Model file for the job. Use its own axes, mm. A direction names the side the tool comes from. Round coordinates to 2 decimals unless told otherwise and drop trailing zeros. Loops run counter-clockwise (first coordinate to the right, second up) from the corner with the lowest first, then second, coordinate; pieces in that order, holes last. Notation, with made-up numbers: M -29,-34.75 L -18,-34.75 A13 ccw -18,-22.75 Z; hole C 72.25,34 d5. An arc over 180 degrees is marked long. Answer in a Markdown table with one row per item.
from build123d import *

# Parameters (mm, degrees)
F0_R      = 30
F1_DEPTH  = 20
F2_R      = 4
F3_DEPTH  = 30
F4_R      = 21.9
F5_DEPTH  = 5
F6_SIZE   = 2
F7_R      = 20
F7_R_2    = 19.9
F8_DEPTH  = 42
F9_R      = 21.9
F9_R_2    = 20
F10_DEPTH = 3
F12_DEPTH = 70
F13_R     = 4
F14_DEPTH = 30.0010001


with BuildPart() as f1:
    # F0 (on Top) → F1 (new body)
    with BuildSketch(Plane.XY):
        Circle(F0_R)
    extrude(amount=F1_DEPTH)

    # F2 (on Front) → F3 (cut)
    with BuildSketch(Plane.XZ):
        with Locations((0, 10.1209855556)):
            Circle(F2_R)
    extrude(amount=F3_DEPTH, mode=Mode.SUBTRACT)

    # F4 (on face) → F5 (join)
    with BuildSketch(Plane.XY.offset(20)):
        Circle(F4_R)
    extrude(amount=F5_DEPTH)

    # F6
    f6_edges = [f1.edges().sort_by_distance(p)[0] for p in [
        (-21.9, 0, 25),
    ]]
    chamfer(f6_edges, length=F6_SIZE)

    # F7 (on face) → F8 (join)
    with BuildSketch(Plane.XY.offset(25)):
        Circle(F7_R)
        Circle(F7_R_2, mode=Mode.SUBTRACT)
        Circle(F7_R_2)
    extrude(amount=F8_DEPTH)

    # F9 (on face) → F10 (join)
    with BuildSketch(Plane.XY.offset(67)):
        Circle(F9_R)
        Circle(F9_R_2, mode=Mode.SUBTRACT)
        Circle(F9_R_2)
    extrude(amount=F10_DEPTH)

    # F11 (on face) → F12 (cut)
    with BuildSketch(Plane.XY.offset(70)):
        with BuildLine():
            Line((18.9816207227, 3.9478135966), (16.0207605252, 3.9478135966))
            ThreePointArc((16.0207605252, 3.9478135966), (-16.5, 0), (16.0207605252, -3.9478135966))
            Line((16.0207605252, -3.9478135966), (18.9816207227, -3.9478135966))
            Line((18.9816207227, -3.9478135966), (18.9816207227, 3.9478135966))
        make_face()
    extrude(amount=-F12_DEPTH, mode=Mode.SUBTRACT)

    # F13 (on Right) → F14 (cut, through all)
    with BuildSketch(Plane.YZ):
        with Locations((0, 8.8561634937)):
            Circle(F13_R)
    extrude(amount=F14_DEPTH, mode=Mode.SUBTRACT)


solid = f1.part
1. Tool access for faces 4 (the flat face through (2, -22, 20)), 5 (the flat face through (10, -18, 67)), 6 (the flat face through (17, -3.948, 40)): list every direction of +Z, -Z, +X, -X, +Y, -Y with a clear straight run to the whole face (end or side of a thin tool).
Verdict:
| item | result |
|---|---|
| face 4 | +Z |
| face 5 | none |
| face 6 | +Z, -Z |
2. Wall check: probe 1 along Z at (x, y) = (-22, -15); probe 2 along Z at (x, y) = (0, -24.25); probe 3 along Z at (x, y) = (21, 0). Give the ranges that are in metal, low to high.
Verdict:
| item | result |
|---|---|
| probe 1 | z = 0 to 20 |
| probe 2 | z = 0 to 6.12, 14.12 to 20 |
| probe 3 | z = 0 to 4.86, 12.86 to 23.9, 67 to 70 |
3. Mould opens along Y. For faces 1 (the flat face through (13, -13, 0)), 2 (the cylindrical face through (-4.336, -19.524, 45.706)), 3 (the flat face through (18, 3.948, 40)) say: +Y half, -Y half, draft (parallel to the pull), parting line (faces both ways), or undercut.
Verdict:
| item | result |
|---|---|
| face 1 | draft |
| face 2 | parting line |
| face 3 | undercut |
4. Saw through at C-C (z = 43). Write the cut outline in (x, y), and give its area (3 significant figures).
Verdict:
| item | result |
|---|---|
| outline | C 0,0 d40; hole M 16.02,-3.95 L 18.98,-3.95 L 18.98,3.95 L 16.02,3.95 A16.5 ccw long Z |
| area | 380 mm² |
5. Pin check, flat tips, straight feed: pin 1 (1.5 mm diameter, centred on x = 17.5, z = 41, fed in from -Y); pin 2 (13 mm diameter, centred on x = 7, y = -5, fed in from -Z); pin 3 (1 mm diameter, centred on x = 1.5, z = 22, fed in from -Y); pin 4 (8.5 mm diameter, centred on y = 1.5, z = 5.5, fed in from -X). Stop position of each tip, or through.
Verdict:
| item | result |
|---|---|
| pin 1 | stops at y = -10.93 |
| pin 2 | passes through |
| pin 3 | stops at y = -21.88 |
| pin 4 | stops at x = -30 |
6. Saw through at D-D (y = -24). Write the cut outline in (x, z), and give its area (3 significant figures).
Verdict:
| item | result |
|---|---|
| outline | M -18,0 L 18,0 L 18,20 L -18,20 Z; hole C 0,10.12 d8 |
| area | 670 mm² |
7. Saw through at A-A (x = 0). Write the cut outline in (y, z), and give its area (3 significant figures).
Verdict:
| item | result |
|---|---|
| outline | M -30,0 L -16.5,0 L -16.5,6.12 L -30,6.12 Z; M -30,14.12 L -16.5,14.12 L -16.5,70 L -21.9,70 L -21.9,67 L -20,67 L -20,25 L -19.9,25 L -21.9,23 L -21.9,20 L -30,20 Z; M 16.5,0 L 30,0 L 30,20 L 21.9,20 L 21.9,23 L 19.9,25 L 20,25 L 20,67 L 21.9,67 L 21.9,70 L 16.5,70 Z |
| area | 808 mm² |
8. Saw through at B-B (y = 0). Write the cut outline in (x, z).
Verdict:
| item | result |
|---|---|
| outline | M -30,0 L -16.5,0 L -16.5,70 L -21.9,70 L -21.9,67 L -20,67 L -20,25 L -19.9,25 L -21.9,23 L -21.9,20 L -30,20 Z; M 18.98,0 L 30,0 L 30,4.86 L 18.98,4.86 Z; M 18.98,12.86 L 30,12.86 L 30,20 L 21.9,20 L 21.9,23 L 19.9,25 L 20,25 L 20,67 L 21.9,67 L 21.9,70 L 18.98,70 Z |
